Design review of the part shown in the three views and the two pictorial views. Dimensions are in mm from the part's minimum x, y and z. A direction names the side the tool comes from. Give positions to 0.01 mm unless a question says otherwise; leave off trailing zeros. Loops run counter-clockwise (first coordinate to the right, second up) from the corner with the lowest first, then second, coordinate; pieces in that order, holes last. Notation, with made-up numbers: (-28.75, 17) -> (13.25, 17) arc R27 ccw to (13.25, 34) -> close; hole circle Ø10 at (62, 69). An arc over 180 degrees is marked (long way). Use CSV: the item, a comma, the result in double quotes. Start each with the question number.
Item 1: The part is to be moulded in two halves that separate along Z. For the marked faces 1, 2, 3 and 4, say which applies: +Z half, -Z half, draft (parallel to the pull), parting line (faces both ways), or undercut.
Item 2: Wall thickness on line 1 along X through (y, z) = (4.25, 5); line 2 along X through (y, z) = (4.1, 53); line 3 along X through (y, z) = (10, 31): over which ranges is each line inside the solid? List them lowest first. Write a range as from..to.
Item 3: For the marked faces 5, 6 and 7, list the 3-axis set-ups (+Z, -Z, +X, -X, +Y, -Y) from which the entire face can be reached by the end or side of a thin tool; tool diameter is ignored.
Item 4: We need section D-D (z = 23.5). State the section outline as (x, y) points.
Item 5: We need section C-C (x = 19.5). State the section outline as (y, z) points.
Item 6: We need section B-B (y = 10.25). Count the separate pieces of the cut face and the enclosed holes in it, plus the area to 3 significant figures.
Item 7: Clearance check with flat-ended pins moving along their axes: pin 1 (1.4 mm diameter, centred on y = 2, z = 52, fed in from +X); pin 2 (2.5 mm diameter, centred on y = 1.5, z = 51.5, fed in from -X); pin 3 (6 mm diameter, centred on x = 36, z = 15, fed in from +Y). State where each tip first meets the part, or that it passes through.
Item 8: We need section A-A (y = 1.25). State the section outline as (x, z) points (1 decimal).
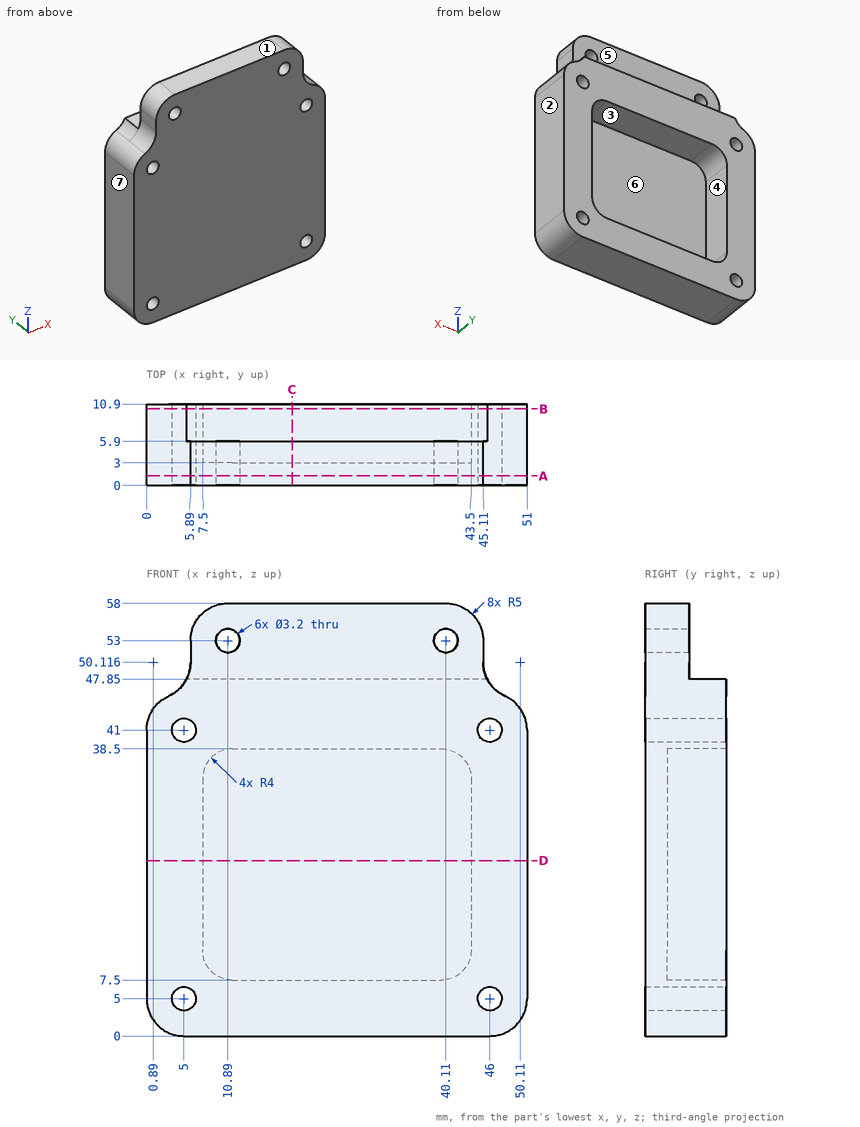
Results found:
1,face 1,"+Z half"
1,face 2,"draft"
1,face 3,"undercut"
1,face 4,"undercut"
2,line 1,"0..3.4, 6.6..44.4, 47.6..51"
2,line 2,"5.89..9.29, 12.49..38.51, 41.71..45.11"
2,line 3,"0..7.5, 43.5..51"
3,face 5,"+Z, +X, -X, +Y"
3,face 6,"+Y"
3,face 7,"+Z, -Z, -X, +Y, -Y"
4,outline,"(0, 0) -> (51, 0) -> (51, 10.9) -> (43.5, 10.9) -> (43.5, 3) -> (7.5, 3) -> (7.5, 10.9) -> (0, 10.9) -> close"
5,outline,"(0, 0) -> (10.9, 0) -> (10.9, 7.5) -> (3, 7.5) -> (3, 38.5) -> (10.9, 38.5) -> (10.9, 47.85) -> (5.9, 47.85) -> (5.9, 58) -> (0, 58) -> close"
6,separate pieces,"1"
6,enclosed holes,"5"
6,area,"1,270 mm²"
7,pin 1,"x = 45.11"
7,pin 2,"x = 5.89"
7,pin 3,"y = 3"
8,outline,"(0, 5) arc R5 ccw to (5, 0) -> (46, 0) arc R5 ccw to (51, 5) -> (51, 41) arc R5 ccw to (48.1, 45.6) arc R5 cw to (45.1, 50.1) -> (45.1, 53) arc R5 ccw to (40.1, 58) -> (10.9, 58) arc R5 ccw to (5.9, 53) -> (5.9, 50.1) arc R5 cw to (2.9, 45.6) arc R5 ccw to (0, 41) -> close; hole circle Ø3.2 at (5, 5); hole circle Ø3.2 at (5, 41); hole circle Ø3.2 at (10.9, 53); hole circle Ø3.2 at (40.1, 53); hole circle Ø3.2 at (46, 5); hole circle Ø3.2 at (46, 41)"
